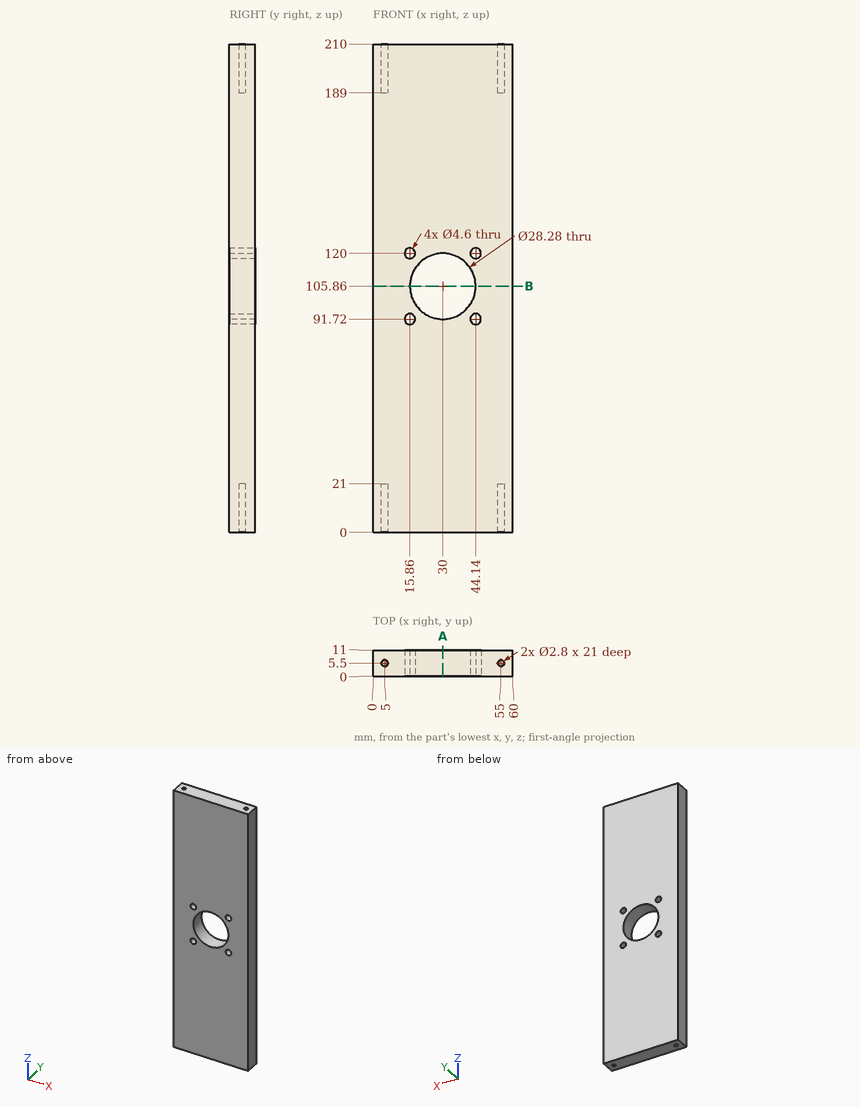
Answer from the drawing. Dimensions are ordinates in mm from the lowest x, y and z of the part. Coordinates: 2 decimals unless noted, no trailing zeros. Order: outer loops, then holes, each group sorted by start corner. A loop starts at its lowest first (then second) coordinate and runs counter-clockwise, first axis right, second up. Notation, with made-up numbers: (-3, 78) -> (33, 78) arc R18 cw to (33, 93) -> close; hole circle Ø4 at (-35.5, 16.25). An arc over 180 degrees is marked (long way). Answer as a JSON object with one key per item and string values.
1) A cutting plane is placed at A-A, the plane x = 30. Determine the outline of the cut face in (y, z), plus the area to 3 significant figures.
Model answer:
{"outline": "(0, 0) -> (11, 0) -> (11, 91.72) -> (0, 91.72) -> close; (0, 120) -> (11, 120) -> (11, 210) -> (0, 210) -> close", "area": "2,000 mm²"}
2) Consider line 1 along Z through (x, y) = (43, 7.5); line 2 along X through (y, z) = (8.5, 105.86); line 3 along Y through (x, z) = (55, 199.75). Determine where each line is inside the solid, lowest interval first. Write a range as from..to.
Model answer:
{"line 1": "z = 0..89.72, 93.72..100.3, 111.42..118, 122..210", "line 2": "x = 0..15.86, 44.14..60", "line 3": "y = 0..4.1, 6.9..11"}
3) A cutting plane is placed at B-B, the plane z = 105.86. Determine the outline of the cut face in (x, y), plus the area to 3 significant figures.
Model answer:
{"outline": "(0, 0) -> (15.86, 0) -> (15.86, 11) -> (0, 11) -> close; (44.14, 0) -> (60, 0) -> (60, 11) -> (44.14, 11) -> close", "area": "349 mm²"}
4) Each of these flat-tipped pins is pushed along its axis until it touches: pin 1 (4 mm diameter, centred on x = 44.14, z = 120, fed in from -Y); pin 2 (0.8 mm diameter, centred on x = 55, y = 6, fed in from +Z); pin 3 (1.7 mm diameter, centred on x = 55, y = 5.5, fed in from -Z). Where does it stop, or does it pass through?
Model answer:
{"pin 1": "passes through", "pin 2": "stops at z = 189", "pin 3": "stops at z = 21"}
